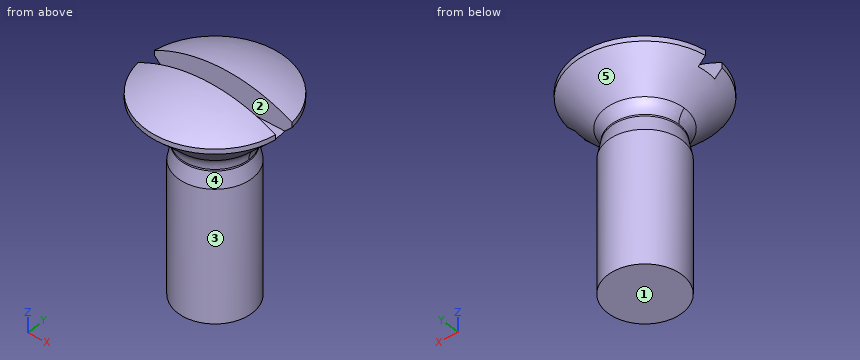
Autodesk Inventor part; units mm, degrees
ref_plane "WorkPlane11" through (0, 0, 0) normal (0, 0, 1) x (1, 0, 0)
ref_plane "Work Plane2" through (0, 0, -5.7) normal (0, 0, 1) x (1, 0, 0)
ref_plane "WorkPlane9" through (0, 0, 8.3) normal (0, 0, 1) x (1, 0, 0)
ref_plane "WorkPlane11" through (0, 0, 0) normal (0, 0, 1) x (1, 0, 0)
ref_plane "Work Plane2" through (0, 0, -5.7) normal (0, 0, 1) x (1, 0, 0)
ref_plane "WorkPlane9" through (0, 0, 8.3) normal (0, 0, 1) x (1, 0, 0)
sketch "Sketch1" plane through (0, 0, 0) normal (0, 0, 1) x (1, 0, 0)
  point P0 (0, 0)
sketch "Sketch2" plane through (0, 0, 0) normal (0, 0, 1) x (1, 0, 0)
  circle A0 centre (0, 0) radius 2.75
  dimension "d2" = 5.5
extrude "Extrusion1" add sketch "Sketch2" against normal blind 0.75
sketch "Sketch3" plane through (0, 0, -0.75) normal (0, 0, -1) x (-1, 0, 0)
  circle A0 centre (0, 0) radius 3
  circle A1 centre (0, 0) radius 2.75 construction
  dimension "d8" = 6
extrude "Extrusion2" add sketch "Sketch3" along normal blind 11.95
sketch "Sketch4" plane through (0, 0, 0) normal (0, 0, 1) x (1, 0, 0)
  circle A0 centre (0, 0) radius 5.65
  circle A1 centre (0, 0) radius 2.75 construction
  dimension "d12" = 11.3
extrude "Extrusion3" add sketch "Sketch4" along normal blind 3.3
sketch "Sketch5" plane through (0, 0, 0) normal (0, 1, 0) x (-1, 0, 0)
  line L0 (5.65, 0) -> (2.75, 0)
  line L1 (5.65, 2.9) -> (5.65, 0)
  line L2 (2.75, 0) -> (5.65, 2.9)
  line L3 (-5.65, 0) -> (5.65, 0) construction
  line L4 (0, -7.6493) -> (0, 5.8993)
  line L5 (0, -10.359) -> (0, 8.609)
  line L6 (5.65, 0) -> (5.65, 3.3)
  line L7 (-4.75, 0) -> (4.75, 0)
  line L8 (2.75, 0) -> (2.75, -0.75)
  dimension "d17" = 45
revolve "Revolution1" cut sketch "Sketch5" angle 360 about axis through (0, 0, -7.6493) along (0, 0, 1)
sketch "Sketch6" plane through (0, 0, 0) normal (0, 1, 0) x (-1, 0, 0)
  line L0 (0, 3.3) -> (0, 4.7133)
  line L1 (0, 3.3) -> (5.65, 3.3)
  arc A0 (5.65, 3.3) -> (0, 4.7133) centre (0, -7.2867) ccw
  line L2 (-5.65, 3.3) -> (5.65, 3.3) construction
  line L3 (0, -7.6493) -> (0, 5.8993)
  line L4 (0, -10.359) -> (0, 8.609)
  line L5 (5.65, 2.9) -> (5.65, 3.3)
  arc A1 (0, 4.7133) -> (-5.65, 3.3) centre (0, -7.2867) ccw
  dimension "d20" = 12
  dimension "d24" = 5.65
revolve "Revolution2" add sketch "Sketch6" angle 360 about axis through (0, 0, -7.6493) along (0, 0, 1)
fillet "Fillet1" radius 1.5 2 edges at (0, 2.75, 0) (0, -2.75, 0)
chamfer "Chamfer1" distance 1.25 distance2 0.25 1 edges at (3, 0, -0.75) measured on face at (-2.9903, -0.2414, -8.7167)
sketch "Sketch8" plane through (0, 0, 0) normal (0, 1, 0) x (-1, 0, 0)
  line L0 (-5.65, 4.7133) -> (5.65, 4.7133)
  line L1 (5.65, 4.7133) -> (5.65, 2.3133)
  line L2 (5.65, 2.3133) -> (-5.65, 2.3133)
  line L3 (-5.65, 2.3133) -> (-5.65, 4.7133)
  arc A0 (5.65, 3.3) -> (-5.65, 3.3) centre (0, -7.2867) ccw
  line L4 (-5.65, 2.9) -> (-5.65, 3.3)
  line L5 (5.65, 2.9) -> (5.65, 3.3)
  dimension "msp_d31" = 2.4
extrude "Extrusion4" cut sketch "Sketch8" against normal mid plane 1.6
thread "Thread1"
ref_plane "MSC_PF1" through (0, 0, 0) normal (1, 0, 0) x (0, 1, 0)
ref_plane "MSC_PT1" through (-5.65, 0, 2.9) normal (0, 0, -1) x (-1, 0, 0)
equation "\"d28\" = r"
equation "\"d29\" = msp_x"
equation "\"d30\" = 0.25 * PTC"
equation "\"d3\" = -msp_x + ParA"
equation "\"d8\" = NND"
equation "\"d9\" = msp_x - ParK + NLG - ParA"
equation "\"d12\" = Dk"
equation "\"d13\" = ParK"
equation "\"msp_d31\" = ParT"
equation "\"msp_d32\" = ParN"
equation "\"d2\" = 0.5 * PTC + msp_mdtds"
equation "\"d20\" = rf"
equation "\"d24\" = 0.5 * Dk"
equation "\"PTC\" = 1"
equation "\"NND\" = 6"
equation "\"msp_x\" = 1.25 * PTC"
equation "\"NLG\" = 16"
equation "\"msp_mdtds\" = NND - PTC"
equation "\"ParK\" = 3.3"
equation "\"ParN\" = 1.6"
equation "\"ParT\" = 2.4"
equation "\"r\" = 1.5"
equation "\"prf_c\" = 0"
equation "\"ParA\" = 2"
equation "\"Dk\" = 11.3"
equation "\"rf\" = 12"
equation "\"ParF\" = 1.4"
equation "\"THREADDIA\" = NND"
equation "\"PG\" = 1.2345"
equation "\"TEMPLATE\" = 1.2345"
properties part number "ISO 2010 - M6x16" material "Stainless Steel, 440C"
Verification items for the finished model (mm, model axes). Face numbers are marked on the shaded views. A direction names the side the tool comes from. Give positions to 0.01 mm unless a question says otherwise; leave off trailing zeros. Write each loop counter-clockwise with the first axis right and the second up, starting at its lowest first coordinate (ties: lowest second). Pieces come first, ordered by that corner, then holes.
(1) Material ranges on line 1 (Z direction, x = 1.75, y = 0.25); line 2 (Z direction, x = 0.75, y = -4.75); line 3 (X direction, y = 1.25, z = -5.5), recorded low to high.
(2) Access from +Z, -Z, +X, -X, +Y, -Y to the whole of each face (thin tool, end or side, straight path). Record for the marked faces 1 and 2.
(3) Cross-section at A-A (z = -9). Enter the section's corners in (x, y), plus the area to 3 significant figures.
(4) Gauge pin test, flat ends, axial feed: pin 1 (1.5 mm diameter, centred on x = -4, z = -5, fed in from +Y); pin 2 (0.7 mm diameter, centred on x = 0.5, z = 4, fed in from +Y); pin 3 (1 mm diameter, centred on x = 2.5, z = -5, fed in from +Y); pin 4 (4 mm diameter, centred on y = 4, z = -9.5, fed in from +X). Record the tip position at first contact, or that the pin passes through.
(5) Mould release check, pull along Z, two halves, no side actions. Record for the marked faces 3, 4 and 5: +Z half, -Z half, draft (parallel to the pull), parting line (faces both ways), or undercut.
Worked out:
1. line 1: z = -12.7 to 2.31
1. line 2: z = 2.06 to 3.71
1. line 3: x = -2.73 to 2.73
2. face 1: -Z, +X, -X, +Y, -Y
2. face 2: +Z, +X, -X
3. outline: circle Ø6 at (0, 0)
3. area: 28.3 mm2
4. pin 1: passes through
4. pin 2: stops at y = 4.91
4. pin 3: stops at y = 2.24
4. pin 4: stops at x = 2.24
5. face 3: draft
5. face 4: undercut
5. face 5: -Z half
